from build123d import *

# Parameters (mm, degrees)
SKETCH_1_R          = 13.85
EXTRUDE_1_DEPTH     = 32.6
SKETCH_2_R          = 18.5
EXTRUDE_2_DEPTH     = 30.5
SKETCH_3_R          = 6
EXTRUDE_3_DEPTH     = 6
SKETCH_4_R          = 3
EXTRUDE_4_DEPTH     = 15
CUT_EXTRUDE_START   = -12
CUT_EXTRUDE_1_DEPTH = 12
SKETCH_6_R          = 1.5
CUT_EXTRUDE_2_DEPTH = 3.5
SKETCH_7_R          = 5
EXTRUDE_5_DEPTH     = 2.6
EXTRUDE_START       = -2.6
SKETCH_8_R          = 1.15
EXTRUDE_6_DEPTH     = 8.5
SKETCH_9_W          = 0.4
SKETCH_9_H          = 2.3
EXTRUDE_7_DEPTH     = 6.9


with BuildPart() as part:
    # ｽｹｯﾁ1 → ﾎﾞｽ - 押し出し1 (new body)
    with BuildSketch(Plane.XY):
        Circle(SKETCH_1_R)
    extrude(amount=EXTRUDE_1_DEPTH)

    # ｽｹｯﾁ2 → ﾎﾞｽ - 押し出し2 (add)
    with BuildSketch(Plane.XY.offset(32.6)):
        with Locations(Location((0, 0, 0), (0, 0, 180))):
            Circle(SKETCH_2_R)
    extrude(amount=EXTRUDE_2_DEPTH)

    # ｽｹｯﾁ3 → ﾎﾞｽ - 押し出し3 (add)
    with BuildSketch(Plane.XY.offset(63.1)):
        with Locations((0, 7)):
            Circle(SKETCH_3_R)
    extrude(amount=EXTRUDE_3_DEPTH)

    # ｽｹｯﾁ4 → ﾎﾞｽ - 押し出し4 (add)
    with BuildSketch(Plane.XY.offset(69.1)):
        with Locations((0, 7)):
            Circle(SKETCH_4_R)
    extrude(amount=EXTRUDE_4_DEPTH)

    # ｽｹｯﾁ5 → ｶｯﾄ - 押し出し1 (cut)
    with BuildSketch(Plane.XY.offset(84.1).offset(CUT_EXTRUDE_START)):
        with BuildLine():
            Line((-1.658312395, 9.5), (1.658312395, 9.5))
            ThreePointArc((1.658312395, 9.5), (0, 10), (-1.658312395, 9.5))
        make_face()
    extrude(amount=CUT_EXTRUDE_1_DEPTH, mode=Mode.SUBTRACT)

    # ｽｹｯﾁ6 → ｶｯﾄ - 押し出し2 (cut)
    with BuildSketch(Plane.XY.offset(63.1)):
        with Locations((-15.5, 0)):
            Circle(SKETCH_6_R)
        with Locations((-7.75, 13.423393759)):
            Circle(SKETCH_6_R)
        with Locations((7.75, 13.423393759)):
            Circle(SKETCH_6_R)
        with Locations((15.5, 0)):
            Circle(SKETCH_6_R)
        with Locations((7.75, -13.423393759)):
            Circle(SKETCH_6_R)
        with Locations((-7.75, -13.423393759)):
            Circle(SKETCH_6_R)
    extrude(amount=-CUT_EXTRUDE_2_DEPTH, mode=Mode.SUBTRACT)

    # ｽｹｯﾁ7 → ﾎﾞｽ - 押し出し5 (add)
    with BuildSketch(Plane(origin=(0, 0, 0), x_dir=(-1, 0, 0), z_dir=(0, 0, -1))):
        Circle(SKETCH_7_R)
    extrude(amount=EXTRUDE_5_DEPTH)

    # ｽｹｯﾁ8 → ﾎﾞｽ - 押し出し6 (add)
    with BuildSketch(Plane(origin=(0, 0, -2.6), x_dir=(-1, 0, 0), z_dir=(0, 0, -1)).offset(EXTRUDE_START)):
        with Locations(Location((0, 0, 0), (0, 0, 180))):
            Circle(SKETCH_8_R)
    extrude(amount=EXTRUDE_6_DEPTH)

    # ｽｹｯﾁ9 → ﾎﾞｽ - 押し出し7 (add)
    with BuildSketch(Plane(origin=(0, 0, 0), x_dir=(-1, 0, 0), z_dir=(0, 0, -1))):
        with Locations((11.65, 0)):
            Rectangle(SKETCH_9_W, SKETCH_9_H)
        with Locations((-11.65, 0)):
            Rectangle(SKETCH_9_W, SKETCH_9_H)
    extrude(amount=EXTRUDE_7_DEPTH)


solid = part.part
Here's how the part is built. I have some questions about the finished solid (model axes, mm). A direction names the side the tool comes from. Coordinates: 2 decimals unless noted, no trailing zeros. Loops run counter-clockwise (first coordinate to the right, second up) from the corner with the lowest first, then second, coordinate; pieces in that order, holes last. Notation, with made-up numbers: (-5, 2.25) -> (48, 2.25) arc R6 cw to (48, 8.25) -> close; hole circle Ø5 at (44.25, -23). An arc over 180 degrees is marked (long way). Use one line per item in the form item = value. Start each with the question number.
(1) If we section it at A-A (x = 0): Please give me the cut outline in (y, z).
(2) Please list where these lines run through material, in increasing order: line 1 along Y through (x, z) = (7, 62); line 2 along Y through (x, z) = (-7.75, 61.25); line 3 along Z through (x, y) = (2.5, -3).
(3) If we section it at C-C (z = 48): Please give me the cut outline in (x, y), then the cut area to 3 significant figures.
(4) If we section it at D-D (x = -8): Please give me the cut outline in (y, z).
(5) On a 3-axis mill with a long thin cutter (end or side, diameter ignored), from which of +Z, -Z, +X, -X, +Y, -Y can I reach the whole of each face in a straight line? I mean faces 1 (the face through (-17, 0, 61)), 2 (the face through (0, 9.5, 78)), 3 (the face through (-11.45, 0, -3)). Say none if no direction works.
(6) Will these pins go through, and if not, where does the flat tip stop? pin 1 (0.7 mm diameter, centred on y = 0.5, z = -5, fed in from -X); pin 2 (2.5 mm diameter, centred on x = 15, y = -0.5, fed in from +Z); pin 3 (3 mm diameter, centred on y = -12, z = 55.5, fed in from +X); pin 4 (14 mm diameter, centred on x = 7, y = 2, fed in from -Z).
(7) We'd pull the mould along X, two halves only. Please class faces 4 (the face through (-11.85, 0, -3)), 5 (the face through (11.85, 0, -3)), 6 (the face through (1, 10, 69.1)), 7 (the face through (8, -13, 59.6)): pulls with the +X half, pulls with the -X half, needs draft (parallel to the pull), parting line crosses it, or undercut.
Verdict:
q1.outline = (-18.5, 32.6) -> (-13.85, 32.6) -> (-13.85, 0) -> (-5, 0) -> (-5, -2.6) -> (-1.15, -2.6) -> (-1.15, -8.5) -> (1.15, -8.5) -> (1.15, -2.6) -> (5, -2.6) -> (5, 0) -> (13.85, 0) -> (13.85, 32.6) -> (18.5, 32.6) -> (18.5, 63.1) -> (13, 63.1) -> (13, 69.1) -> (10, 69.1) -> (10, 72.1) -> (9.5, 72.1) -> (9.5, 84.1) -> (4, 84.1) -> (4, 69.1) -> (1, 69.1) -> (1, 63.1) -> (-18.5, 63.1) -> close
q2.line_1 = -17.12 to -14.72, -12.12 to 12.12, 14.72 to 17.12
q2.line_2 = -16.8 to -14.92, -11.92 to 11.92, 14.92 to 16.8
q2.line_3 = -2.6 to 63.1
q3.outline = circle Ø37 at (0, 0)
q3.area = 1,080 mm²
q4.outline = (-16.68, 32.6) -> (-11.31, 32.6) -> (-11.31, 0) -> (11.31, 0) -> (11.31, 32.6) -> (16.68, 32.6) -> (16.68, 63.1) -> (14.9, 63.1) -> (14.9, 59.6) -> (11.94, 59.6) -> (11.94, 63.1) -> (-11.94, 63.1) -> (-11.94, 59.6) -> (-14.9, 59.6) -> (-14.9, 63.1) -> (-16.68, 63.1) -> close
q5.face_1 = +Z
q5.face_2 = +Z, +X, -X, +Y
q5.face_3 = -Z, +Y, -Y
q6.pin_1 = -11.85
q6.pin_2 = 63.1
q6.pin_3 = 15.23
q6.pin_4 = -8.5
q7.face_4 = pulls with the -X half
q7.face_5 = pulls with the +X half
q7.face_6 = needs draft
q7.face_7 = undercut
